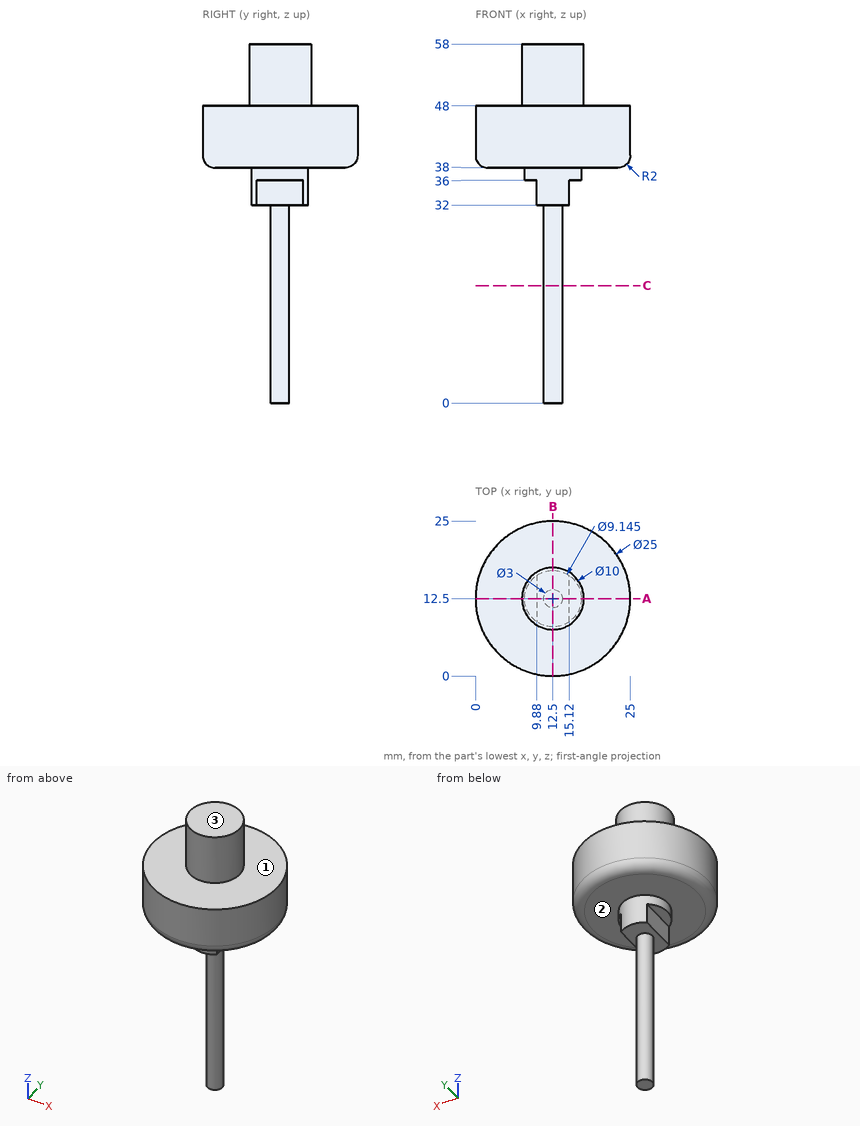
Print and shaded views of the part. All mm, measured from the part's lowest x, y and z. A direction names the side the tool comes from. Coordinates: 2 decimals unless noted, no trailing zeros. Loops run counter-clockwise (first coordinate to the right, second up) from the corner with the lowest first, then second, coordinate; pieces in that order, holes last. Notation, with made-up numbers: M -5,42 L 0,42 A31 cw 0,81 Z; hole C -28.75,64 d9. An arc over 180 degrees is marked long. Use a Markdown table: item, result. Add a question column.
Q1. Probe L1, parallel to Z at x = 22.5, y = 10.75; L2, parallel to X at y = 12.5, z = 14; L3, parallel to X at y = 5.75, z = 40. List the from-to ranges inside material, lowest first.
Q2. Which spindle directions (+Z, -Z, +X, -X, +Y, -Y) get a long thin tool onto all of the face, cutting with end or side? Do the marked faces 1, 2 and 3. Say none if no direction does.
Q3. Cut at C-C (z = 19). Write the cut outline in (x, y).
Q4. Cut at B-B (x = 12.5). Write the cut outline in (y, z), and give its area (3 significant figures).
Q5. Pin check, flat tips, straight feed: P1, Ø1.6, axis at x = 16, y = 12.5, coming from the -Z side; P2, Ø2, axis at y = 12.5, z = 34.5, coming from the +X side; P3, Ø5, axis at x = 9.5, y = 20.5, coming from the +Z side; P4, Ø12, axis at x = 19.5, y = 14.5, coming from the -Z side. Stop position of each tip, or through.
Q6. Cut at A-A (y = 12.5). Write the cut outline in (x, z).
Worked out:
| question | item | result |
|---|---|---|
| 1 | L1 | z = 38 to 48 |
| 1 | L2 | x = 11 to 14 |
| 1 | L3 | x = 1.98 to 23.02 |
| 2 | face 1 | +Z |
| 2 | face 2 | -Z |
| 2 | face 3 | +Z, +X, -X, +Y, -Y |
| 3 | outline | C 12.5,12.5 d3 |
| 4 | outline | M 0,40 A2 ccw 2,38 L 7.93,38 L 7.93,32 L 11,32 L 11,0 L 14,0 L 14,32 L 17.07,32 L 17.07,38 L 23,38 A2 ccw 25,40 L 25,48 L 17.5,48 L 17.5,58 L 7.5,58 L 7.5,48 L 0,48 Z |
| 4 | area | 499 mm2 |
| 5 | P1 | stops at z = 36 |
| 5 | P2 | stops at x = 15.12 |
| 5 | P3 | stops at z = 48 |
| 5 | P4 | stops at z = 0 |
| 6 | outline | M 0,40 A2 ccw 2,38 L 7.93,38 L 7.93,36 L 9.88,36 L 9.88,32 L 11,32 L 11,0 L 14,0 L 14,32 L 15.12,32 L 15.12,36 L 17.07,36 L 17.07,38 L 23,38 A2 ccw 25,40 L 25,48 L 17.5,48 L 17.5,58 L 7.5,58 L 7.5,48 L 0,48 Z |
